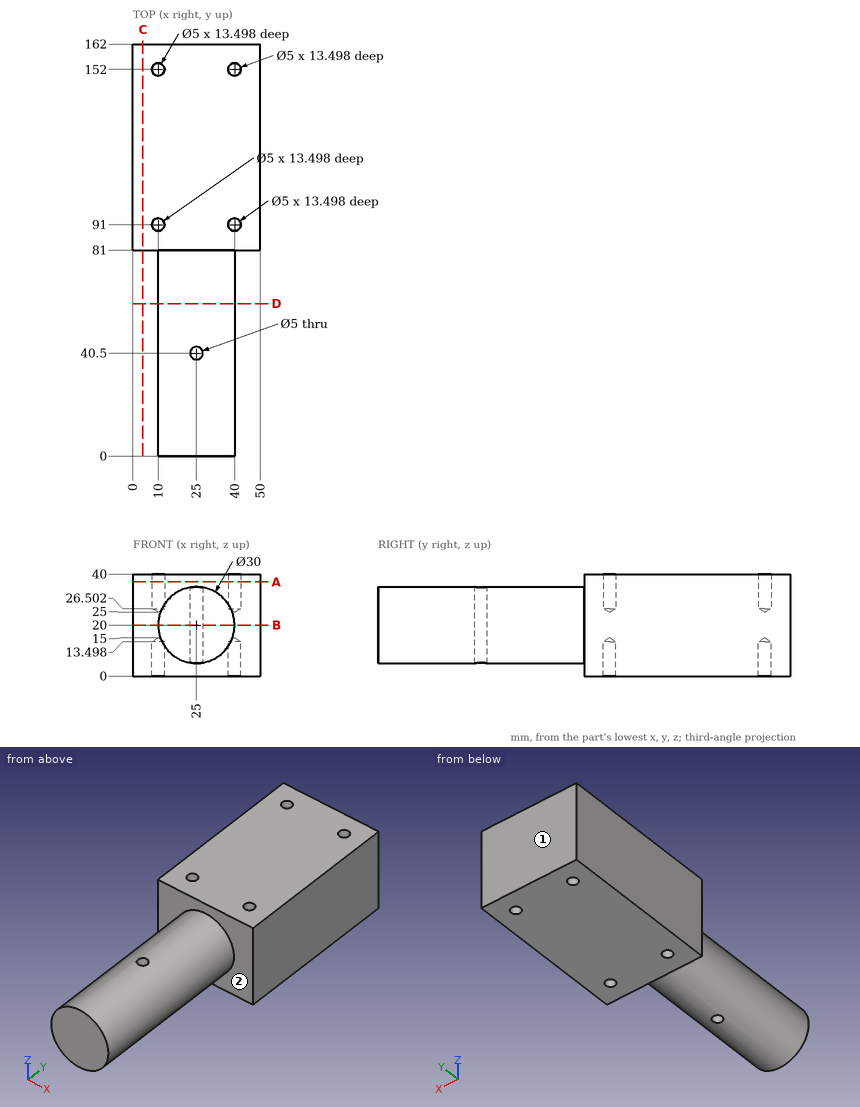
Answer from the drawing. Dimensions are ordinates in mm from the lowest x, y and z of the part. A direction names the side the tool comes from. Coordinates: 2 decimals unless noted, no trailing zeros. Order: outer loops, then holes, each group sorted by start corner. A loop starts at its lowest first (then second) coordinate and runs counter-clockwise, first axis right, second up. Notation, with made-up numbers: M 59.25,4.25 L 107.25,4.25 A21 ccw 107.25,30.25 Z; hole C 33.5,55 d1. An arc over 180 degrees is marked long. Put each result on its own line as item: value. Start each with the question number.
Item 1: Section B-B, the plane z = 20 is taken. Determine the outline of the cut face in (x, y), plus the area to 3 significant figures.
Item 2: Section C-C, the plane x = 4 is taken. Determine the outline of the cut face in (y, z).
Item 3: Section A-A, the plane z = 37 is taken. Determine the outline of the cut face in (x, y), plus the area to 3 significant figures.
Item 4: For the marked faces 1 and 2, determine the directions among +Z, -Z, +X, -X, +Y, -Y from which every point of the face is accessible in a straight line to the end or side of a thin tool.
Item 5: Section D-D, the plane y = 60 is taken. Determine the outline of the cut face in (x, z), plus the area to 3 significant figures.
Item 6: Consider probe 1 along Y at (x, z) = (10, 32); probe 2 along Y at (x, z) = (25, 28.5); probe 3 along Y at (x, z) = (31, 4.5). Determine where each line is inside the solid, lowest interval first. Write a range as [from, to].
Item 7: Given pin 1 Ø3 at (x, y) = (40, 91) entering from +Z; pin 2 Ø8 at (x, y) = (40, 152) entering from +Z; pin 3 Ø1.5 at (x, z) = (44.5, 18) entering from -Y; pin 4 Ø1 at (y, z) = (71.5, 14) entering from +X (1 decimal), each flat-ended and moving along its own axis, determine where each tip first touches the part or whether it passes through.
Computed:
1. outline: M 0,81 L 10,81 L 10,0 L 40,0 L 40,81 L 50,81 L 50,162 L 0,162 Z; hole C 25,40.5 d5
1. area: 6,460 mm2
2. outline: M 81,0 L 162,0 L 162,40 L 81,40 Z
3. outline: M 0,81 L 50,81 L 50,162 L 0,162 Z; hole C 10,91 d5; hole C 10,152 d5; hole C 40,91 d5; hole C 40,152 d5
3. area: 3,970 mm2
4. face 1: +Z, -Z, +X, -X, +Y
4. face 2: -Y
5. outline: C 25,20 d30
5. area: 707 mm2
6. probe 1: y = [81, 88.5], [93.5, 149.5], [154.5, 162]
6. probe 2: y = [0, 38], [43, 162]
6. probe 3: y = [81, 162]
7. pin 1: stops at z = 25.9
7. pin 2: stops at z = 40
7. pin 3: stops at y = 81
7. pin 4: stops at x = 39
